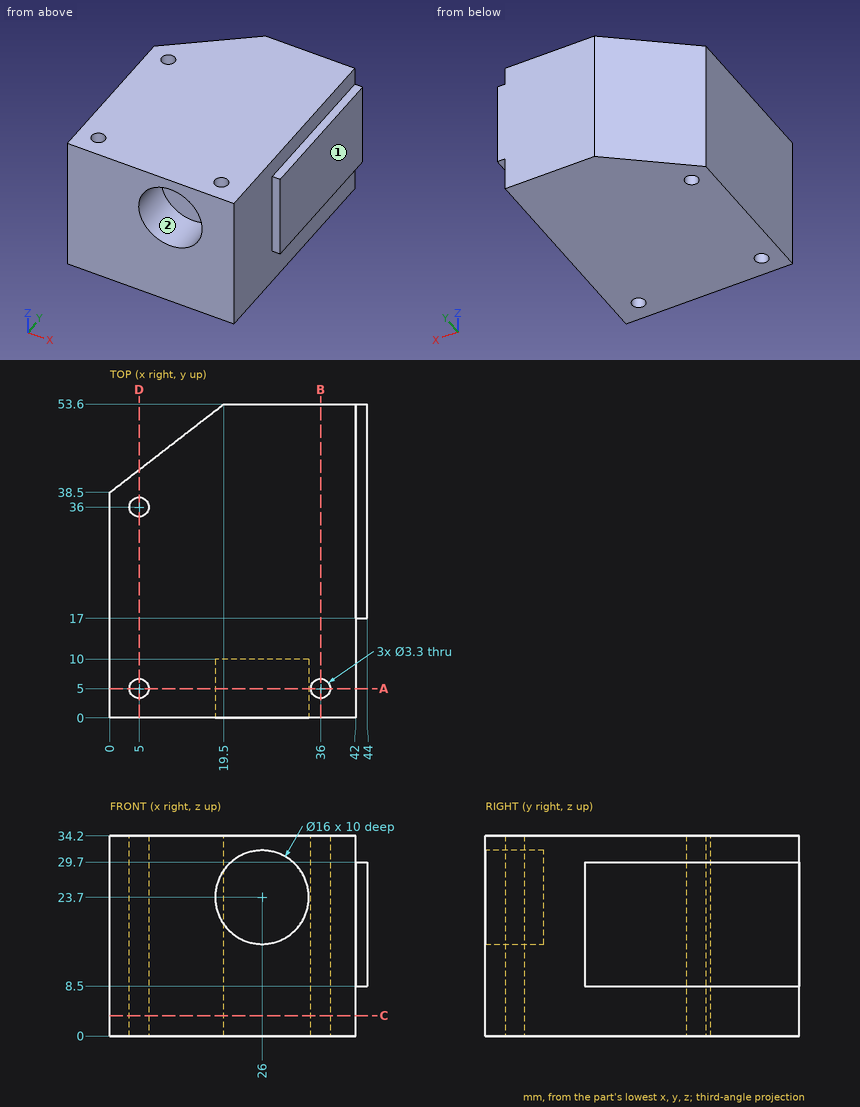
Verification items for this drawing (mm, ordinates from the low corner). A direction names the side the tool comes from. Round coordinates to 2 decimals unless told otherwise and drop trailing zeros. Loops run counter-clockwise (first coordinate to the right, second up) from the corner with the lowest first, then second, coordinate; pieces in that order, holes last. Notation, with made-up numbers: (32.25, 5.25) -> (51.25, 5.25) arc R20 ccw to (51.25, 38.25) -> close; hole circle Ø10 at (18, 34.5). An arc over 180 degrees is marked (long way). Answer in a Markdown table with one row per item.
Q1. Sectioned sample at D-D on x = 5. Enter the section's corners in (y, z), then the cut area to 3 significant figures.
Data:
| item | result |
|---|---|
| outline | (0, 0) -> (3.35, 0) -> (3.35, 34.2) -> (0, 34.2) -> close; (6.65, 0) -> (34.35, 0) -> (34.35, 34.2) -> (6.65, 34.2) -> close; (37.65, 0) -> (42.37, 0) -> (42.37, 34.2) -> (37.65, 34.2) -> close |
| area | 1,220 mm^2 |
Q2. Go/stop test with flat-tipped pins: P1, Ø2.5, axis at x = 5, y = 36, coming from the -Z side; P2, Ø0.6, axis at x = 43.5, y = 29.5, coming from the +Z side; P3, Ø1, axis at x = 43, z = 24.5, coming from the -Y side. Record where each tip stops, or that it passes through.
Data:
| item | result |
|---|---|
| P1 | passes through |
| P2 | stops at z = 29.7 |
| P3 | stops at y = 17 |
Q3. Set-up check for the marked faces 1 and 2: record each of +Z, -Z, +X, -X, +Y, -Y from which the full face is reachable in a straight line by a thin tool's end or side.
Data:
| item | result |
|---|---|
| face 1 | +Z, -Z, +X, +Y, -Y |
| face 2 | -Y |
Q4. Sectioned sample at C-C on z = 3.5. Enter the section's corners in (x, y), then the cut area to 3 significant figures.
Data:
| item | result |
|---|---|
| outline | (0, 0) -> (42, 0) -> (42, 53.6) -> (19.5, 53.6) -> (0, 38.5) -> close; hole circle Ø3.3 at (5, 5); hole circle Ø3.3 at (5, 36); hole circle Ø3.3 at (36, 5) |
| area | 2,080 mm^2 |
Q5. Sectioned sample at A-A on y = 5. Enter the section's corners in (x, z).
Data:
| item | result |
|---|---|
| outline | (0, 0) -> (3.35, 0) -> (3.35, 34.2) -> (0, 34.2) -> close; (6.65, 0) -> (34.35, 0) -> (34.35, 34.2) -> (6.65, 34.2) -> close; (37.65, 0) -> (42, 0) -> (42, 34.2) -> (37.65, 34.2) -> close; hole circle Ø16 at (26, 23.7) |
Q6. Sectioned sample at B-B on x = 36. Enter the section's corners in (y, z), then the cut area to 3 significant figures.
Data:
| item | result |
|---|---|
| outline | (0, 0) -> (3.35, 0) -> (3.35, 34.2) -> (0, 34.2) -> close; (6.65, 0) -> (53.6, 0) -> (53.6, 34.2) -> (6.65, 34.2) -> close |
| area | 1,720 mm^2 |
Q7. Thickness scan on L1, parallel to X at y = 6, z = 23.7; L2, parallel to Y at x = 5, z = 21; L3, parallel to Y at x = 27.5, z = 18.5. Record the ranges inside material, lowest first.
Data:
| item | result |
|---|---|
| L1 | x = 0 to 3.69, 6.31 to 18, 34 to 34.69, 37.31 to 42 |
| L2 | y = 0 to 3.35, 6.65 to 34.35, 37.65 to 42.37 |
| L3 | y = 10 to 53.6 |
